from build123d import *


with BuildPart() as part:
    # Çizim1 → Döndür2 (revolve)
    with BuildSketch(Plane.XY, mode=Mode.PRIVATE) as d_nd_r2_sk:
        with BuildLine():
            Line((0, 0), (0, 21.5))
            Line((0, 21.5), (11, 21.5))
            Line((11, 21.5), (11, 15.5))
            Line((11, 15.5), (30, 15.5))
            Line((30, 15.5), (30, 32))
            Line((30, 32), (39, 32))
            Line((39, 32), (39, 15.5))
            Line((39, 15.5), (73, 15.5))
            Line((73, 15.5), (98, 12.5))
            Line((98, 12.5), (98, 7))
            Line((98, 7), (106, 7))
            Line((106, 7), (106, 12))
            Line((106, 12), (109, 12))
            Line((109, 12), (109, 7))
            ThreePointArc((109, 7), (111, 6.236067977), (113, 7))
            Line((113, 7), (135.5, 7))
            ThreePointArc((135.5, 7), (136.673723702, 3.590797936), (137, 0))
            Line((137, 0), (0, 0))
        make_face()
    revolve(d_nd_r2_sk.sketch.rotate(Axis((0, 0, 0), (1, 0, 0)), 90), axis=Axis((0, 0, 0), (1, 0, 0)))


solid = part.part
Here's how the part is built. I have some questions about the finished solid (model axes, mm). A direction names the side the tool comes from. Round coordinates to 2 decimals unless told otherwise and drop trailing zeros. Write each loop counter-clockwise with the first axis right and the second up, starting at its lowest first coordinate (ties: lowest second). Pieces come first, ordered by that corner, then holes.
1. Will these pins go through, and if not, where does the flat tip stop? pin 1 Ø4 at (x, z) = (57.5, 3.5) entering from -Y; pin 2 Ø4 at (x, y) = (15, 19) entering from -Z; pin 3 Ø19 at (y, z) = (-3.5, 4.5) entering from +X; pin 4 Ø6 at (x, y) = (90.5, -7) entering from -Z.
2. Suppose I cut it at D-D (x = 15.5). List the corners of the cut face in (y, z) for me.
3. Suppose I cut it at A-A (x = 79). List the corners of the cut face in (y, z) for me.
4. Suppose I cut it at B-B (y = -24). List the corners of the cut face in (x, z) for me, and give its area (3 significant figures).
5. For faces 1 (the cylindrical face through (56.238, -15.368, -2.018)), 2 (the flat face through (30, -8, -14)), 3 (the cylindrical face through (5.577, -21.317, -2.799)), which set-ups out of +Z, -Z, +X, -X, +Y, -Y let a thin tool reach every point of the face, with its end or its side?
6. If we mould it in two halves opening along X, with no side actions, what happens to faces 4 (the cylindrical face through (34.56, 31.24, -6.94)), 5 (the flat face through (11, -11.2, 11)), 6 (the flat face through (39, -8, 14))? For each: released by +X, released by -X, zero draft, split by the parting line, or undercut.
7. I need wall thicknesses on L1, parallel to X at y = -10.5, z = -13; L2, parallel to X at y = 5, z = 10; L3, parallel to X at y = -28, z = -9. Which ranges of each line are inside material? Lowest first, please.
Answer sheet:
1. pin 1: stops at y = -15.43
1. pin 2: passes through
1. pin 3: stops at x = 137.01
1. pin 4: stops at z = -12.86
2. outline: circle Ø31 at (0, 0)
3. outline: circle Ø29.56 at (0, 0)
4. outline: (30, -21.17) - (39, -21.17) - (39, 21.17) - (30, 21.17) - close
4. area: 381 mm2
5. face 1: +X
5. face 2: none
5. face 3: -X
6. face 4: zero draft
6. face 5: undercut
6. face 6: released by +X
7. L1: x = 0 to 11, 30 to 39
7. L2: x = 0 to 98, 106 to 109
7. L3: x = 30 to 39
